Could you check a few things on this model? Use its own coordinates, in mm. A direction names the side the tool comes from. Give positions to 0.01 mm unless a question says otherwise; leave off trailing zeros. Loops run counter-clockwise (first coordinate to the right, second up) from the corner with the lowest first, then second, coordinate; pieces in that order, holes last. Notation, with made-up numbers: (-27.75, 76.25) -> (-18.75, 76.25) arc R13 cw to (-18.75, 96.25) -> close; hole circle Ø8 at (6.5, -14.5). An arc over 180 degrees is marked (long way). Write each question's results on one line, items separated by ' | '. Start each with the question number.
Q1. Will these pins go through, and if not, where does the flat tip stop? P1, Ø0.6, axis at y = -3, z = 3.5, coming from the +X side; P2, Ø1.6, axis at y = -3, z = 2.5, coming from the -X side; P3, Ø1, axis at y = -3, z = 4, coming from the +X side; P4, Ø1.6, axis at y = -3.5, z = 3, coming from the -X side.
Q2. If I drill on line 1 along Y through (x, z) = (-3.5, 1.5); line 2 along X through (y, z) = (-6.5, 5.25); line 3 along X through (y, z) = (-9, 5.25), over which ranges is the centre line in solid material (lowest first)?
Q3. Which directions (+Z, -Z, +X, -X, +Y, -Y) give clear straight access to the entire face, cutting with the end or side of a thin tool? Please do faces 4 (the face through (-95.287, -3, 3)), 5 (the face through (-75.225, -20.449, 3.451)), 6 (the face through (-56, -37.546, 3)).
Q4. We'd pull the mould along X, two halves only. Please class faces 1 (the face through (-87.44, -33.2, 3.45)), 2 (the face through (-15.75, -25.11, 3.45)), 3 (the face through (-26.37, -9.82, 3.55)): released by +X, released by -X, zero draft, split by the parting line, or undercut.
Q5. If we section it at B-B, the plane y = -33: List the corners of the cut face in (x, z) for me.
Q6. If we section it at A-A, the plane z = 5.5: Give the number of separate pieces and of enclosed holes in the cut face, plus the area to 3 significant figures.
Q7. If we section it at C-C, the plane x = -42.5: List the corners of the cut face in (y, z) for me, plus the area to 3 significant figures.
from build123d import *

# Parameters (mm, degrees)
F0_R        = 1.5
F1_DEPTH    = 7
F2_R        = 3.99999
F3_T1_DEPTH = 37
F4_W        = 20
F4_H        = 7
F5_DEPTH    = 6
F6_W        = 1.5
F6_H        = 7
F7_DEPTH    = 2


# Not quite as in the source:
# - a fillet or chamfer that OpenCascade refuses, or shapes differently, is made with other operations: its cross-section is extruded or revolved along the edge and cut away or added
# - a fillet or chamfer is up to 0.001 mm smaller than in the source, because OpenCascade refuses the exact size


with BuildPart() as f1:
    # F0 (on Top) → F1 (new body)
    with BuildSketch(Plane.XY):
        Polygon((-79.2163482308, -9.9173756316), (-95.3576945582, -9.9173756316), (-95.3576945582, -28.9785558952), (-79.2939967774, -37.5458613783), (-31.2939967774, -37.5458613783), (4.9152223427, -8.5784860822), (-2.401850828, 0.5678553812), (-21.1427022546, -14.4248257601), (-26.1402626351, -8.1778752846), (-32.3872131106, -13.175435665), (-27.3896527302, -19.4223861405), (-31.2939967774, -22.5458613783), (-71.2939967774, -22.5458613783), (-79.2678481488, -18.2931406469), align=None)
        with Locations((-26.7649576826, -13.8001307126)):
            Circle(F0_R, mode=Mode.SUBTRACT)
        with Locations((-3.3164724251, -7.6638418965)):
            Circle(F0_R, mode=Mode.SUBTRACT)
    extrude(amount=F1_DEPTH)

    # F2 (radius 4 in the source; OpenCascade refuses exactly that, so slightly less here)
    f2_edges = [f1.edges().sort_by_distance(p)[0] for p in [
        (-26.140263, -8.177875, 3.5),
        (-32.387213, -13.175436, 3.5),
    ]]
    fillet(f2_edges, radius=F2_R)

    # F3: fillet of radius 6 on 2 edges, made by hand

    # F3_s2 → F3_t1 (cut)
    with BuildSketch(Plane.XY.offset(-15)):
        with BuildLine():
            ThreePointArc((-7.0870636847, -3.1803149041), (-2.6763042429, -1.9022253527), (1.3463194573, -4.1173574755))
            Line((1.3463194573, -4.1173574755), (-2.401850828, 0.5678553812))
            Line((-2.401850828, 0.5678553812), (-7.0870636847, -3.1803149041))
        make_face()
        with BuildLine():
            ThreePointArc((1.1670520574, -3.8932732256), (2.4451416088, -8.3040326673), (0.2300094861, -12.3266563675))
            Line((0.2300094861, -12.3266563675), (4.9152223427, -8.5784860822))
            Line((4.9152223427, -8.5784860822), (1.1670520574, -3.8932732256))
        make_face()
    extrude(amount=F3_T1_DEPTH, mode=Mode.SUBTRACT)

    # F4 (on face) → F5 (join)
    with BuildSketch(Plane(origin=(0, -9.9173756316, 0), x_dir=(-1, 0, 0), z_dir=(0, 1, 0))):
        with Locations((87.2870213945, 3.5)):
            Rectangle(F4_W, F4_H)
    extrude(amount=F5_DEPTH)

    # F6 (on face) → F7 (join)
    with BuildSketch(Plane(origin=(0, -3.9173756316, 0), x_dir=(-1, 0, 0), z_dir=(0, 1, 0))):
        with Locations((78.0370213945, 3.5)):
            Rectangle(F6_W, F6_H)
        with Locations((81.0370213945, 3.5)):
            Rectangle(F6_W, F6_H)
        with Locations((84.0370213945, 3.5)):
            Rectangle(F6_W, F6_H)
        with Locations((87.0370213945, 3.5)):
            Rectangle(F6_W, F6_H)
        with Locations((90.0370213945, 3.5)):
            Rectangle(F6_W, F6_H)
        with Locations((93.0370213945, 3.5)):
            Rectangle(F6_W, F6_H)
        with Locations((96.0370213945, 3.5)):
            Rectangle(F6_W, F6_H)
    extrude(amount=F7_DEPTH)


solid = f1.part
Final values:
1) P1: stops at x = 0.55 | P2: stops at x = -96.79 | P3: stops at x = 0.78 | P4: stops at x = -97.29
2) line 1: y = -15.31 to -9.15, -6.18 to -1.87 | line 2: x = -97.29 to -77.29, -11.24 to -4.26, -2.37 to 2.37 | line 3: x = -97.29 to -77.29, -14.36 to -4, -2.63 to 2.33
3) face 4: +Z, -Z, +Y | face 5: +Z, -Z | face 6: +Z, -Z, +X, -X, -Y
4) face 1: released by -X | face 2: released by +X | face 3: undercut
5) outline: (-87.82, 0) -> (-25.61, 0) -> (-25.61, 7) -> (-87.82, 7) -> close
6) separate pieces: 1 | enclosed holes: 2 | area: 1,770 mm²
7) outline: (-37.55, 0) -> (-22.55, 0) -> (-22.55, 7) -> (-37.55, 7) -> close | area: 105 mm²
